Here's how the part is built. I have some questions about the finished solid (model axes, mm). Coordinates: 2 decimals unless noted, no trailing zeros. Loops run counter-clockwise (first coordinate to the right, second up) from the corner with the lowest first, then second, coordinate; pieces in that order, holes last. Notation, with made-up numbers: (65, 47) - (110, 47) arc R18 cw to (110, 80) - close; hole circle Ø8 at (-36, 21.25). An arc over 180 degrees is marked (long way). Use a Markdown table: item, result.
Solid Edge part; units mm, degrees
sketch "Sketch1" plane through (0, 0, 0) normal (1, 0, 0) x (0, 1, 0)
  line L0 (0, 0) -> (53.8724, 0)
sketch "Sketch2" plane through (0, 0, 0) normal (0, -1, 0) x (1, 0, 0)
  line L0 (-25.4, -14.6647) -> (0, -29.3294)
  line L1 (0, -29.3294) -> (25.4, -14.6647)
  line L2 (25.4, -14.6647) -> (25.4, 14.6647)
  line L3 (25.4, 14.6647) -> (0, 29.3294)
  line L4 (0, 29.3294) -> (-25.4, 14.6647)
  line L5 (-25.4, 14.6647) -> (-25.4, -14.6647)
sweep "Protrusion_1" add profiles "Sketch2" path "Sketch1"
Q1. I want a section at A-A, the plane y = 27. Write out the boundary of the cut face in (x, z), then the cut area to 3 significant figures.
Check values:
| item | result |
|---|---|
| outline | (-25.4, -14.66) - (0, -29.33) - (25.4, -14.66) - (25.4, 14.66) - (0, 29.33) - (-25.4, 14.66) - close |
| area | 2,230 mm^2 |
Q2. Please list where these lines run through material, in increasing order: L1, parallel to Z at x = -5, y = 47; L2, parallel to X at y = 12, z = -17.5; L3, parallel to Z at x = 21, y = 22. Write a range as from..to.
Check values:
| item | result |
|---|---|
| L1 | -26.44..26.44 |
| L2 | -20.49..20.49 |
| L3 | -17.21..17.21 |
Q3. Will these pins go through, and if not, where does the flat tip stop? P1, Ø2, axis at x = -6, y = 9, coming from the -Z side; P2, Ø8, axis at x = -5, y = 27, coming from the -Z side.
Check values:
| item | result |
|---|---|
| P1 | z = -26.44 |
| P2 | z = -28.75 |
Q4. I want a section at C-C, the plane z = -18.5. Write out the boundary of the cut face in (x, y), then the cut area to 3 significant figures.
Check values:
| item | result |
|---|---|
| outline | (-18.76, 0) - (18.76, 0) - (18.76, 53.87) - (-18.76, 53.87) - close |
| area | 2,020 mm^2 |
Q5. I want a section at B-B, the plane x = 19.5. Write out the boundary of the cut face in (y, z).
Check values:
| item | result |
|---|---|
| outline | (0, -18.07) - (53.87, -18.07) - (53.87, 18.07) - (0, 18.07) - close |
